Verification items for the finished model (mm, model axes). Round coordinates to 2 decimals unless told otherwise and drop trailing zeros. Loops run counter-clockwise (first coordinate to the right, second up) from the corner with the lowest first, then second, coordinate; pieces in that order, holes last. Notation, with made-up numbers: (47, 21.5) -> (66, 21.5) arc R31 cw to (66, 54.5) -> close; hole circle Ø2 at (32, 69). An arc over 180 degrees is marked (long way). Write item = value, one per line. Start each with the question number.
```python
from build123d import *

# Parameters (mm, degrees)
F1_DEPTH = 2.3622
F2_R     = 1.016


with BuildPart() as f1:
    # F0 (on Front) → F1 (new body)
    with BuildSketch(Plane.XZ):
        with BuildLine():
            Line((-1.27, -14.4221906796), (-1.27, 14.4221906796))
            ThreePointArc((-1.27, 14.4221906796), (-14.478, 0), (-1.27, -14.4221906796))
        make_face()
    extrude(amount=-F1_DEPTH)

    # F2
    f2_edges = [f1.edges().sort_by_distance(p)[0] for p in [
        (-14.478, 0, 0),
        (-1.27, 0, 0),
        (-14.478, 2.3622, 0),
        (-1.27, 2.3622, 0),
    ]]
    fillet(f2_edges, radius=F2_R)


solid = f1.part
```
(1) Depth check by flat-ended pin: pin 1 Ø1 at (y, z) = (1.5, -6.5) entering from +X. Enter the tip coordinate at first touch or a pass-through.
(2) Scan lines: line 1 (X direction, y = 1.35, z = -1.25); line 2 (Z direction, x = -4, y = 1.9); line 3 (X direction, y = 1.8, z = 10.75). Record each from-to range of solid material in increasing order. Write a range as [from, to].
(3) Section check B-B on y = 2.05. Enter the section's corners in (x, z).
(4) Section check C-C on y = 0.35. Enter the section's corners in (x, z).
(5) Section check A-A on z = 0. Enter the section's corners in (x, y), then the cut area to 3 significant figures.
Computed values:
q1.pin_1 = -1.27
q2.line_1 = [-14.42, -1.27]
q2.line_2 = [-13.74, 13.74]
q2.line_3 = [-9.54, -1.38]
q3.outline = (-1.55, -14.11) -> (-1.55, 14.11) arc R14.19 ccw to start
q4.outline = (-1.52, -14.15) -> (-1.52, 14.15) arc R14.23 ccw to start
q5.outline = (-14.48, 1.02) arc R1.02 ccw to (-13.46, 0) -> (-2.29, 0) arc R1.02 ccw to (-1.27, 1.02) -> (-1.27, 1.35) arc R1.02 ccw to (-2.29, 2.36) -> (-13.46, 2.36) arc R1.02 ccw to (-14.48, 1.35) -> close
q5.area = 30.3 mm²
